from build123d import *

# Parameters (mm, degrees)
P_IDAT_VYSUNUT_M1_DEPTH  = 3
SKICA3_R                 = 1
ODEBRAT_VYSUNUT_M1_DEPTH = 3


with BuildPart() as part:
    # Skica1 → Rotovat1 (revolve)
    with BuildSketch(Plane.XY, mode=Mode.PRIVATE) as rotovat1_sk:
        Polygon((1, 5.88592233), (3, 5.88592233), (3, -0.11407767), (2.5, -0.11407767), (2.5, -1.61407767), (3.5, -1.61407767), (3.5, -4.61407767), (3.171296013, -4.61407767), (0.315, -6.61407767), (0.15, -6.61407767), (0.15, -6.11407767), (0.5, -5.76407767), (0.5, -5.11407767), (1, -4.61407767), align=None)
    revolve(rotovat1_sk.sketch.rotate(Axis((0, 5.88592233, 0), (0, -1, 0)), 90), axis=Axis((0, 5.88592233, 0), (0, -1, 0)))

    # Skica2 → Přidat vysunutím1 (add)
    with BuildSketch(Plane(origin=(0, -1.61407767, 0), x_dir=(1, 0, 0), z_dir=(0, 1, 0))):
        Polygon((-4.03408582, 0.243895321), (-2.228262454, -3.371673141), (1.805823366, -3.615568462), (4.03408582, -0.243895321), (2.228262454, 3.371673141), (-1.805823366, 3.615568462), align=None)
    extrude(amount=-P_IDAT_VYSUNUT_M1_DEPTH)

    # Skica3 → Odebrat vysunutím1 (cut)
    with BuildSketch(Plane(origin=(0, -1.61407767, 0), x_dir=(1, 0, 0), z_dir=(0, 1, 0))):
        with Locations(Location((0, 0, 0), (0, 0, 270))):
            Circle(SKICA3_R)
    extrude(amount=-ODEBRAT_VYSUNUT_M1_DEPTH, mode=Mode.SUBTRACT)


solid = part.part
CAD build for the part. Positions are in the model's coordinates, mm. A direction names the side the tool comes from. Coordinates: 2 decimals unless noted, no trailing zeros. Write each loop counter-clockwise with the first axis right and the second up, starting at its lowest first coordinate (ties: lowest second). Pieces come first, ordered by that corner, then holes. Notation, with made-up numbers: (77, 53.25) - (102, 53.25) arc R29 ccw to (102, 73.25) - close; hole circle Ø4 at (52, -25). An arc over 180 degrees is marked (long way). Use a Markdown table: item, result. Add a question column.
Item 1: Band-saw the part on D-D, the plane y = 4.25. Give the cut face in (x, z), and give its area (3 significant figures).
Item 2: Flat gauge pins, fed straight in: pin 1 (1.6 mm diameter, centred on x = 0, z = 0, fed in from +Y); pin 2 (3 mm diameter, centred on y = 3, z = -1, fed in from -X); pin 3 (4 mm diameter, centred on y = -4.5, z = -2, fed in from -X); pin 4 (2 mm diameter, centred on x = 1.5, z = 1.5, fed in from -Y). Where does each tip first touch, or does it go through?
Item 3: Drill centre lines: L1, parallel to Z at x = 0.5, y = -4.5; L2, parallel to X at y = -6.25, z = 0; L3, parallel to X at y = -2.5, z = 0. Where is each one in solid material? Low to high. Write a range as from..to.
Item 4: Band-saw the part on C-C, the plane x = 0. Give the cut face in (y, z) (3 decimals), and give its area (3 significant figures).
Item 5: Band-saw the part on B-B, the plane y = -0.25. Give the cut face in (x, z), and give its area (3 significant figures).
Item 6: Band-saw the part on A-A, the plane z = 0. Give the cut face in (x, y) (3 decimals), and give its area (3 significant figures).
Item 7: Mould opens along X. For faces 6 (the face through (3, -1.614, 0)), 7 (the face through (1, 1, 0)), 8 (the face through (2.904, -3.093, 1.953)), 9 (the face through (0.44, -6.52, -0.1)) say: pulls with the +X half, pulls with the -X half, needs draft (parallel to the pull), parting line crosses it, or undercut.
Item 8: 3-axis set-ups, long thin cutter, end or side, ignore diameter. For faces 1 (the face through (0.488, -5.435, -0.108)), 2 (the face through (-2, -0.114, -2)), 3 (the face through (-2.904, -3.093, -1.953)), 4 (the face through (-2, -4.614, 3)), 5 (the face through (0.24, -3.09, -3.49)): which of +Z, -Z, +X, -X, +Y, -Y reach the whole face in a straight line?
Numbers:
| question | item | result |
|---|---|---|
| 1 | outline | circle Ø6 at (0, 0); hole circle Ø2 at (0, 0) |
| 1 | area | 25.1 mm2 |
| 2 | pin 1 | y = -4.81 |
| 2 | pin 2 | x = -3 |
| 2 | pin 3 | x = -4.03 |
| 2 | pin 4 | y = -6.05 |
| 3 | L1 | -3.48..-0.87, 0.87..3.54 |
| 3 | L2 | -0.83..-0.15, 0.15..0.83 |
| 3 | L3 | -3.91..-1, 1..3.91 |
| 4 | outline | (-6.614, -0.315) - (-4.614, -3.171) - (-4.614, -3.506) - (-1.614, -3.506) - (-1.614, -2.5) - (-0.114, -2.5) - (-0.114, -3) - (5.886, -3) - (5.886, -1) - (-4.614, -1) - (-5.114, -0.5) - (-5.764, -0.5) - (-6.114, -0.15) - (-6.614, -0.15) - close; (-6.614, 0.15) - (-6.114, 0.15) - (-5.764, 0.5) - (-5.114, 0.5) - (-4.614, 1) - (5.886, 1) - (5.886, 3) - (-0.114, 3) - (-0.114, 2.5) - (-1.614, 2.5) - (-1.614, 3.506) - (-4.614, 3.506) - (-4.614, 3.171) - (-6.614, 0.315) - close |
| 4 | area | 48.7 mm2 |
| 5 | outline | circle Ø5 at (0, 0); hole circle Ø2 at (0, 0) |
| 5 | area | 16.5 mm2 |
| 6 | outline | (-3.912, -4.614) - (-3.171, -4.614) - (-0.315, -6.614) - (-0.15, -6.614) - (-0.15, -6.114) - (-0.5, -5.764) - (-0.5, -5.114) - (-1, -4.614) - (-1, 5.886) - (-3, 5.886) - (-3, -0.114) - (-2.5, -0.114) - (-2.5, -1.614) - (-3.912, -1.614) - close; (0.15, -6.614) - (0.315, -6.614) - (3.171, -4.614) - (3.912, -4.614) - (3.912, -1.614) - (2.5, -1.614) - (2.5, -0.114) - (3, -0.114) - (3, 5.886) - (1, 5.886) - (1, -4.614) - (0.5, -5.114) - (0.5, -5.764) - (0.15, -6.114) - close |
| 6 | area | 51.2 mm2 |
| 7 | face 6 | needs draft |
| 7 | face 7 | undercut |
| 7 | face 8 | pulls with the +X half |
| 7 | face 9 | parting line crosses it |
| 8 | face 1 | +Y |
| 8 | face 2 | none |
| 8 | face 3 | -Z, -X, +Y, -Y |
| 8 | face 4 | -Y |
| 8 | face 5 | -Z, +X, +Y, -Y |
